Check sheet for the drawn part. Datum: minimum x, y, z corner. Units: mm. A direction names the side the tool comes from. Give positions to 0.01 mm unless a question says otherwise; leave off trailing zeros. Loops run counter-clockwise (first coordinate to the right, second up) from the corner with the lowest first, then second, coordinate; pieces in that order, holes last. Notation, with made-up numbers: (20, -0.75) - (35, -0.75) arc R14 ccw to (35, 3.25) - close; hole circle Ø1 at (22, 11.5). An arc over 180 degrees is marked (long way). Use one line per item in the form item = value.
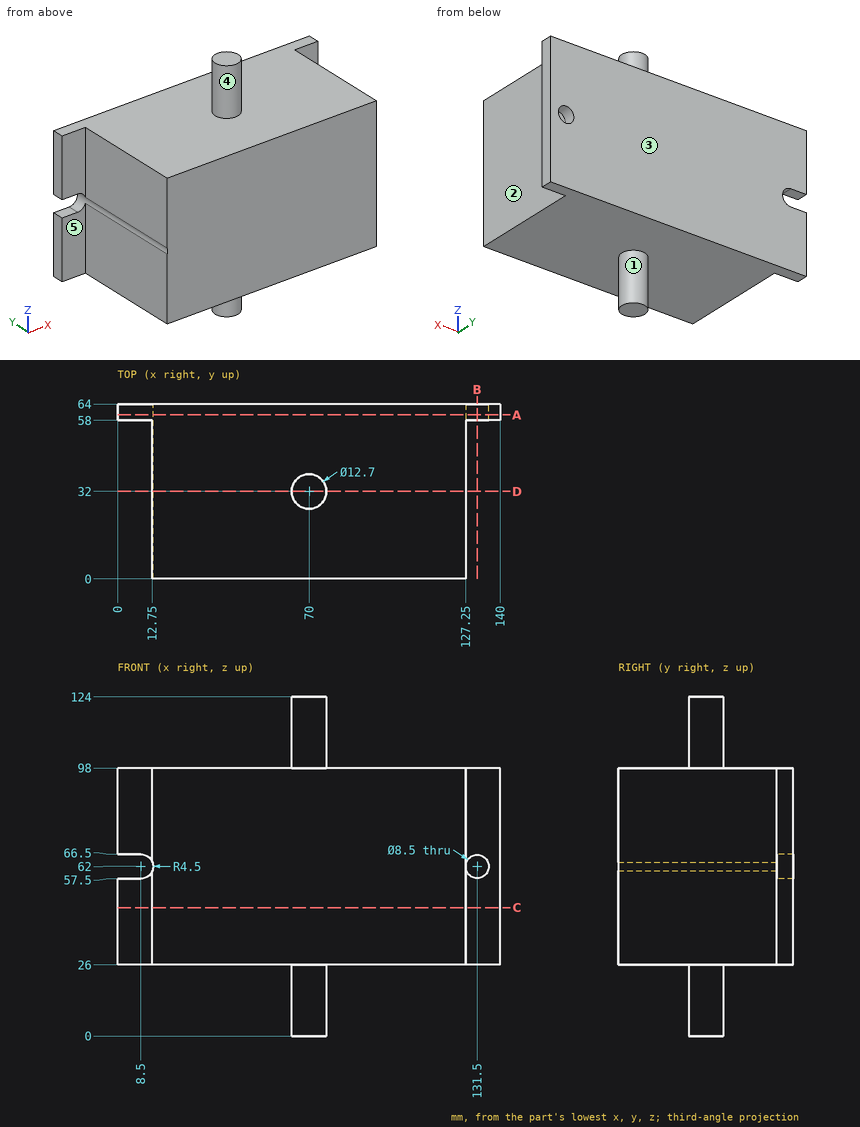
Item 1: Thickness scan on L1, parallel to Z at x = 131.5, y = 62.7; L2, parallel to X at y = 16, z = 90; L3, parallel to Z at x = 24, y = 53. Record the ranges inside material, lowest first.
Answer block:
L1 = 26 to 57.75, 66.25 to 98
L2 = 12.75 to 127.25
L3 = 26 to 98
Item 2: Section check B-B on x = 131.5. Record the boundary of the cut face in (y, z).
Answer block:
outline = (58, 26) - (64, 26) - (64, 57.75) - (58, 57.75) - close; (58, 66.25) - (64, 66.25) - (64, 98) - (58, 98) - close
Item 3: Section check D-D on y = 32. Record the boundary of the cut face in (x, z), then the cut area to 3 significant figures.
Answer block:
outline = (12.75, 26) - (63.65, 26) - (63.65, 0) - (76.35, 0) - (76.35, 26) - (127.25, 26) - (127.25, 98) - (76.35, 98) - (76.35, 124) - (63.65, 124) - (63.65, 98) - (12.75, 98) - (12.75, 63.48) arc R4.5 cw to (12.75, 60.52) - close
area = 8,900 mm2
Item 4: Section check C-C on z = 47. Record the boundary of the cut face in (x, y), then the cut area to 3 significant figures.
Answer block:
outline = (0, 58) - (12.75, 58) - (12.75, 0) - (127.25, 0) - (127.25, 58) - (140, 58) - (140, 64) - (0, 64) - close
area = 7,480 mm2
Item 5: Gauge pin test, flat ends, axial feed: P1, Ø3, axis at x = 109.5, y = 55, coming from the -Z side; P2, Ø19, axis at x = 89, y = 20.5, coming from the +Z side; P3, Ø1, axis at y = 18, z = 65.5, coming from the +X side. Record the tip position at first contact, or that the pin passes through.
Answer block:
P1 = 26
P2 = 98
P3 = 127.25
Item 6: Section check A-A on y = 60. Record the boundary of the cut face in (x, z), then the cut area to 3 significant figures.
Answer block:
outline = (0, 26) - (140, 26) - (140, 98) - (0, 98) - (0, 66.5) - (8.5, 66.5) arc R4.5 cw to (8.5, 57.5) - (0, 57.5) - close; hole circle Ø8.5 at (131.5, 62)
area = 9,910 mm2
Item 7: Access from +Z, -Z, +X, -X, +Y, -Y to the whole of each face (thin tool, end or side, straight path). Record for the marked faces 1, 2, 3, 4 and 5.
Answer block:
face_1 = -Z
face_2 = +Z, -Z, +X, -Y
face_3 = +Z, -Z, +X, -X, +Y
face_4 = +Z
face_5 = +Z, -Z, -X, -Y
